The listing builds one solid part. Answer for the finished solid, in the listing's coordinates (mm). Face numbers are marked on the shaded views. Round coordinates to 2 decimals unless told otherwise and drop trailing zeros. Loops run counter-clockwise (first coordinate to the right, second up) from the corner with the lowest first, then second, coordinate; pieces in that order, holes last. Notation, with made-up numbers: (-0.5, 78.5) -> (44.5, 78.5) arc R20 ccw to (44.5, 107.5) -> close; hole circle Ø7 at (-19.75, -22.75). An arc over 180 degrees is marked (long way). One line per question, with ' | ' between items.
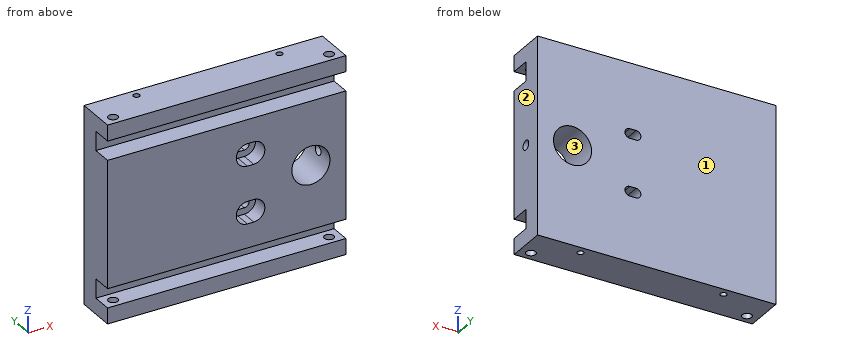
from build123d import *

# Parameters (mm, degrees)
SKETCH1_W             = 150
SKETCH1_H             = 10
BOSS_EXTRUDE1_DEPTH   = 12.5
SKETCH1_H_2           = 80
SKETCH1_R             = 12
BOSS_EXTRUDE1_2_DEPTH = 12.5
BOSS_EXTRUDE1_3_DEPTH = 12.5
BOSS_EXTRUDE2_START   = 12.5
SKETCH1_3_W           = 150
SKETCH1_3_H           = 124
SKETCH1_3_R           = 12
BOSS_EXTRUDE2_DEPTH   = 12.5
SKETCH2_R             = 3
CUT_EXTRUDE1_DEPTH    = 101.468900661
CUT_EXTRUDE2_DEPTH    = 10
SKETCH3_R             = 3
CUT_EXTRUDE3_DEPTH    = 15
SKETCH4_R             = 2
SKETCH4_R_2           = 3
CUT_EXTRUDE4_DEPTH    = 18
CUT_EXTRUDE5_START    = -106
SKETCH4_2_R           = 2
SKETCH4_2_R_2         = 3
CUT_EXTRUDE5_DEPTH    = 18


with BuildPart() as part:
    # Sketch1 → Boss-Extrude1 (new body)
    with BuildSketch(Plane(origin=(0, 0, 0), x_dir=(1, 0, 0), z_dir=(0, 1, 0))):
        with Locations((0, 57)):
            Rectangle(SKETCH1_W, SKETCH1_H)
    extrude(amount=BOSS_EXTRUDE1_DEPTH)



with BuildPart() as body_2:
    # Sketch1 → Boss-Extrude1 2 (new body)
    with BuildSketch(Plane(origin=(0, 0, 0), x_dir=(1, 0, 0), z_dir=(0, 1, 0))):
        Rectangle(SKETCH1_W, SKETCH1_H_2)
        with Locations(Location((53, 0, 0), (0, 0, 270))):
            Circle(SKETCH1_R, mode=Mode.SUBTRACT)
    extrude(amount=BOSS_EXTRUDE1_2_DEPTH)


with BuildPart() as body_3:
    # Sketch1 → Boss-Extrude1 3 (new body)
    with BuildSketch(Plane(origin=(0, 0, 0), x_dir=(1, 0, 0), z_dir=(0, 1, 0))):
        with Locations((0, -57)):
            Rectangle(SKETCH1_W, SKETCH1_H)
    extrude(amount=BOSS_EXTRUDE1_3_DEPTH)


with BuildPart() as part_1:
    add(part.part)

    add(body_2.part)  # Boss-Extrude2 merges body 2

    add(body_3.part)  # Boss-Extrude2 merges body 3
    # Sketch1<3> → Boss-Extrude2 (add)
    with BuildSketch(Plane(origin=(0, 0, 0), x_dir=(1, 0, 0), z_dir=(0, 1, 0)).offset(BOSS_EXTRUDE2_START)):
        Rectangle(SKETCH1_3_W, SKETCH1_3_H)
        with Locations(Location((53, 0, 0), (0, 0, 270))):
            Circle(SKETCH1_3_R, mode=Mode.SUBTRACT)
    extrude(amount=BOSS_EXTRUDE2_DEPTH)

    # Sketch2 → Cut-Extrude1 (cut, through all)
    with BuildSketch(Plane.XZ):
        with Locations((13, -18)):
            Circle(SKETCH2_R)
        with Locations((17, -18)):
            Circle(SKETCH2_R)
        with BuildLine():
            Line((17, -15), (13, -15))
            ThreePointArc((13, -15), (14.070466269, -15.197482923), (15, -15.763932023))
            ThreePointArc((15, -15.763932023), (15.929533731, -15.197482923), (17, -15))
        make_face()
        with BuildLine():
            ThreePointArc((15, -20.236067977), (14.070466269, -20.802517077), (13, -21))
            Line((13, -21), (17, -21))
            ThreePointArc((17, -21), (15.929533731, -20.802517077), (15, -20.236067977))
        make_face()
        with Locations((17, 18)):
            Circle(SKETCH2_R)
        with Locations((13, 18)):
            Circle(SKETCH2_R)
        with BuildLine():
            Line((17, 21), (13, 21))
            ThreePointArc((13, 21), (14.070466269, 20.802517077), (15, 20.236067977))
            ThreePointArc((15, 20.236067977), (15.929533731, 20.802517077), (17, 21))
        make_face()
        with BuildLine():
            ThreePointArc((15, 15.763932023), (14.070466269, 15.197482923), (13, 15))
            Line((13, 15), (17, 15))
            ThreePointArc((17, 15), (15.929533731, 15.197482923), (15, 15.763932023))
        make_face()
    extrude(amount=-CUT_EXTRUDE1_DEPTH, mode=Mode.SUBTRACT)

    # Sketch2<3> → Cut-Extrude2 (cut)
    # profile 1 of 2: a face of its own
    with BuildSketch(Plane.XZ):
        with BuildLine():
            Line((17, 25), (13, 25))
            ThreePointArc((13, 25), (6, 18), (13, 11))
            Line((13, 11), (17, 11))
            ThreePointArc((17, 11), (24, 18), (17, 25))
        make_face()
        with BuildLine():
            ThreePointArc((13, 15), (10, 18), (13, 21))
            Line((13, 21), (17, 21))
            ThreePointArc((17, 21), (19.121320344, 20.121320344), (20, 18))
            ThreePointArc((20, 18), (19.121320344, 15.878679656), (17, 15))
            Line((17, 15), (13, 15))
        make_face(mode=Mode.SUBTRACT)
    # profile 2 of 2: a face of its own
    with BuildSketch(Plane.XZ):
        with BuildLine():
            Line((17, -11), (13, -11))
            ThreePointArc((13, -11), (6, -18), (13, -25))
            Line((13, -25), (17, -25))
            ThreePointArc((17, -25), (24, -18), (17, -11))
        make_face()
        with BuildLine():
            ThreePointArc((13, -21), (10, -18), (13, -15))
            Line((13, -15), (17, -15))
            ThreePointArc((17, -15), (19.121320344, -15.878679656), (20, -18))
            ThreePointArc((20, -18), (19.121320344, -20.121320344), (17, -21))
            Line((17, -21), (13, -21))
        make_face(mode=Mode.SUBTRACT)
    extrude(amount=-CUT_EXTRUDE2_DEPTH, mode=Mode.SUBTRACT)

    # Sketch3 → Cut-Extrude3 (cut)
    with BuildSketch(Plane(origin=(75, 0, 0), x_dir=(0, 0, -1), z_dir=(1, 0, 0))):
        with Locations((0, 12.5)):
            Circle(SKETCH3_R)
    extrude(amount=-CUT_EXTRUDE3_DEPTH, mode=Mode.SUBTRACT)

    # Sketch4 → Cut-Extrude4 (cut)
    with BuildSketch(Plane.XY.offset(62)):
        with Locations((-45, 20)):
            Circle(SKETCH4_R)
        with Locations((45, 20)):
            Circle(SKETCH4_R)
        with Locations((-68, 6)):
            Circle(SKETCH4_R_2)
        with Locations(Location((68, 6, 0), (0, 0, 180))):
            Circle(SKETCH4_R_2)
    extrude(amount=-CUT_EXTRUDE4_DEPTH, mode=Mode.SUBTRACT)

    # Sketch4<2> → Cut-Extrude5 (cut)
    with BuildSketch(Plane.XY.offset(62).offset(CUT_EXTRUDE5_START)):
        with Locations((-45, 20)):
            Circle(SKETCH4_2_R)
        with Locations((45, 20)):
            Circle(SKETCH4_2_R)
        with Locations((-68, 6)):
            Circle(SKETCH4_2_R_2)
        with Locations(Location((68, 6, 0), (0, 0, 180))):
            Circle(SKETCH4_2_R_2)
    extrude(amount=-CUT_EXTRUDE5_DEPTH, mode=Mode.SUBTRACT)


solid = part_1.part
Q1. For a pull along X with two mould halves and no side action, classify the marked faces 1, 2 and 3 as pulls with the +X half, pulls with the -X half, needs draft (parallel to the pull), parting line crosses it, or undercut.
Numbers:
face 1: needs draft | face 2: pulls with the +X half | face 3: undercut
Q2. Given pin 1 Ø6 at (x, z) = (-29.5, -46) entering from -Y; pin 2 Ø1.2 at (x, y) = (-44.5, 19) entering from -Z; pin 3 Ø3 at (x, y) = (45, 20) entering from +Z, each flat-ended and moving along its own axis, determine where each tip first touches the part or whether it passes through.
Numbers:
pin 1: y = 12.5 | pin 2: z = -44 | pin 3: z = 44
Q3. A cutting plane is placed at A-A on x = 53. Give the vertices of the cut face in (y, z).
Numbers:
outline: (0, -62) -> (25, -62) -> (25, -12) -> (0, -12) -> (0, -40) -> (12.5, -40) -> (12.5, -52) -> (0, -52) -> close; (0, 12) -> (25, 12) -> (25, 62) -> (0, 62) -> (0, 52) -> (12.5, 52) -> (12.5, 40) -> (0, 40) -> close
Q4. A cutting plane is placed at B-B on z = 0. Give the vertices of the cut face in (x, y), plus the area to 3 significant figures.
Numbers:
outline: (-75, 0) -> (41, 0) -> (41, 25) -> (-75, 25) -> close; (65, 0) -> (75, 0) -> (75, 9.5) -> (65, 9.5) -> close; (65, 15.5) -> (75, 15.5) -> (75, 25) -> (65, 25) -> close | area: 3,090 mm^2
Q5. A cutting plane is placed at C-C on x = -45. Give the vertices of the cut face in (y, z).
Numbers:
outline: (0, -62) -> (18, -62) -> (18, -44) -> (22, -44) -> (22, -62) -> (25, -62) -> (25, 62) -> (22, 62) -> (22, 44) -> (18, 44) -> (18, 62) -> (0, 62) -> (0, 52) -> (12.5, 52) -> (12.5, 40) -> (0, 40) -> (0, -40) -> (12.5, -40) -> (12.5, -52) -> (0, -52) -> close
Q6. Find the intervals of material crossed by line 1 (Z direction, x = -13.5, y = 4.5); line 2 (Y direction, x = -45, z = -51.25); line 3 (Y direction, x = 68, z = -56.5), in increasing order. Write a range as from..to.
Numbers:
line 1: -62..-52, -40..40, 52..62 | line 2: 12.5..18, 22..25 | line 3: 0..3, 9..25
Q7. A cutting plane is placed at D-D on z = 46. Give the vertices of the cut face in (x, y), plus the area to 3 significant figures.
Numbers:
outline: (-75, 12.5) -> (75, 12.5) -> (75, 25) -> (-75, 25) -> close; hole circle Ø4 at (-45, 20); hole circle Ø4 at (45, 20) | area: 1,850 mm^2
